Source: CAD feature listing. Evaluate the final solid. Frame: model axes, mm. Face numbers are marked on the shaded views. A direction names the side the tool comes from. Coordinates: 2 decimals unless noted, no trailing zeros. Loops run counter-clockwise (first coordinate to the right, second up) from the corner with the lowest first, then second, coordinate; pieces in that order, holes last. Notation, with made-up numbers: M 35.25,88.5 L 46.25,88.5 A12 ccw 46.25,99.5 Z; hole C 48.5,53.5 d5. An arc over 180 degrees is marked long. One line per question, with ' | ' between items. Start each with the question number.
1. Access query for the marked faces 4 and 5. Directions: +Z, -Z, +X, -X, +Y, -Y. A direction counts if a zero-diameter tool reaches every point of the face in a straight line with its end or side. Return the directions, or none.
2. Ray query, probe 1 along Y at (x, z) = (7.75, 0); probe 2 along X at (y, z) = (-1.5, -1.9). Return the intervals inside material, ascending.
3. Section query B-B, the plane x = 13.25. Output: boundary loops of the cut face in (y, z), and give its area (3 significant figures).
4. Pin query (flat end, axial travel): P1, Ø1, axis at x = 7.5, y = 2, coming from the -Z side; P2, Ø2, axis at y = 2, z = -2, coming from the +X side; P3, Ø1.1, axis at x = -1.5, y = -2, coming from the -Z side; P4, Ø0.8, axis at x = -1, y = -1.5, coming from the +Z side. Return the tip coordinate at first contact, or that it passes through.
5. Mould query, pull axis Y, two halves, no side actions, for the marked faces 1, 2 and 3. Classes: pulls with the +Y half, pulls with the -Y half, needs draft (parallel to the pull), parting line crosses it, or undercut.
6. Section query A-A, the plane x = 1.25. Output: boundary loops of the cut face in (y, z).
```python
from build123d import *

# Parameters (mm, degrees)
CUT_EXTRUDE1_DEPTH = 2.1


with BuildPart() as part:
    # Sketch1 → Revolve1 (revolve)
    with BuildSketch(Plane.XY):
        with BuildLine():
            Line((-2.4, 0), (-2.4, 1.4))
            ThreePointArc((-2.4, 1.4), (-2.010193737, 2.178709812), (-1.4, 2.8))
            Line((-1.4, 2.8), (-0.2, 2.8))
            ThreePointArc((-0.2, 2.8), (-0.058578644, 2.741421356), (0, 2.6))
            Line((0, 2.6), (0, 1.6))
            ThreePointArc((0, 1.6), (0.087867966, 1.387867966), (0.3, 1.3))
            Line((0.3, 1.3), (12.1065, 1.3))
            Line((12.1065, 1.3), (12.3065, 1.5))
            Line((12.3065, 1.5), (16.6935, 1.5))
            Line((16.6935, 1.5), (17, 1.1935))
            Line((17, 1.1935), (17, 0))
            Line((17, 0), (-2.4, 0))
        make_face()
    revolve(axis=Axis((17, 0, 0), (-1, 0, 0)))

    # Sketch2 → Cut-Extrude1 (cut)
    with BuildSketch(Plane.ZY.offset(2.4)):
        with BuildLine():
            Line((0.38, -2.014472636), (0.38, -0.975538848))
            ThreePointArc((0.38, -0.975538848), (0.613182892, -0.826946318), (0.88968299, -0.828248869))
            ThreePointArc((0.88968299, -0.828248869), (1.212435563, -0.700000005), (1.162126064, -0.356363644))
            ThreePointArc((1.162126064, -0.356363644), (1.008436863, -6e-09), (1.162126056, 0.356363636))
            ThreePointArc((1.162126056, 0.356363636), (1.212435568, 0.699999995), (0.889683001, 0.828248872))
            ThreePointArc((0.889683001, 0.828248872), (0.613182897, 0.826946316), (0.38, 0.975538848))
            Line((0.38, 0.975538848), (0.38, 2.014472636))
            ThreePointArc((0.38, 2.014472636), (0, 2.05), (-0.38, 2.014472636))
            Line((-0.38, 2.014472636), (-0.38, 0.975538848))
            ThreePointArc((-0.38, 0.975538848), (-0.613182887, 0.826946319), (-0.889682981, 0.828248866))
            ThreePointArc((-0.889682981, 0.828248866), (-1.212435565, 0.700000001), (-1.162126051, 0.356363631))
            ThreePointArc((-1.162126051, 0.356363631), (-1.008436863, -7e-09), (-1.162126061, -0.356363641))
            ThreePointArc((-1.162126061, -0.356363641), (-1.212435561, -0.700000008), (-0.889682979, -0.828248866))
            ThreePointArc((-0.889682979, -0.828248866), (-0.613182886, -0.826946319), (-0.38, -0.975538848))
            Line((-0.38, -0.975538848), (-0.38, -2.014472636))
            ThreePointArc((-0.38, -2.014472636), (0, -2.05), (0.38, -2.014472636))
        make_face()
    extrude(amount=-CUT_EXTRUDE1_DEPTH, mode=Mode.SUBTRACT)

    # Sketch3 → Cut-Revolve1 (revolve, cut)
    with BuildSketch(Plane.XY):
        Polygon((-2.4, 0), (-2.4, 1.4), (-1, 0), align=None)
    revolve(axis=Axis((-1, 0, 0), (-1, 0, 0)), mode=Mode.SUBTRACT)


solid = part.part
```
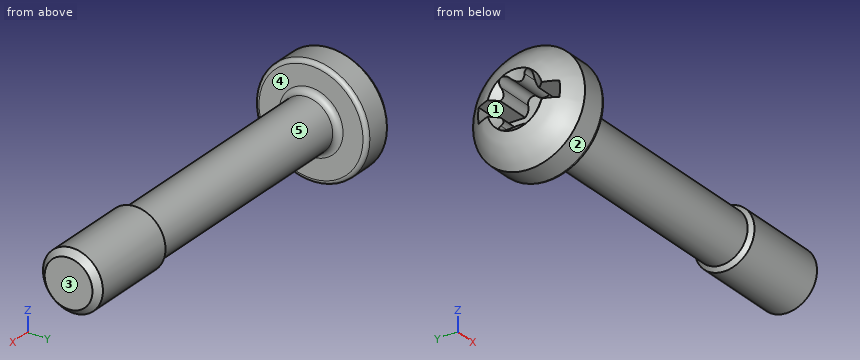
Taken from the geometry:
1) face 4: +X | face 5: none
2) probe 1: -1.3 to 1.3 | probe 2: -1.82 to 0
3) outline: C 0,0 d3 | area: 7.07 mm^2
4) P1: through | P2: x = 0 | P3: z = -2.39 | P4: z = 2.57
5) face 1: undercut | face 2: parting line crosses it | face 3: needs draft
6) outline: C 0,0 d2.6
